from build123d import *

# Parameters (mm, degrees)
F1_DEPTH = 3.24


with BuildPart() as f1:
    # F0 (on Top) → F1 (new body)
    with BuildSketch(Plane.XY):
        Polygon((32.101754, 47.657341), (8.328551, 29.566584), (8.328551, 13.494031), (8.328551, 9.566584), (8.328551, 5.849354), (8.328551, -10.433416), (32.101754, 7.657341), align=None)
        Polygon((8.328551, 9.566584), (8.328551, 13.494031), (1.83994, 13.494031), (1.83994, 5.849354), (8.328551, 5.849354), align=None)
    extrude(amount=F1_DEPTH)


solid = f1.part
Part model, mm, in its own coordinate system. A direction names the side the tool comes from. Coordinates: 2 decimals unless noted, no trailing zeros. Write each loop counter-clockwise with the first axis right and the second up, starting at its lowest first coordinate (ties: lowest second). Pieces come first, ordered by that corner, then holes. Notation, with made-up numbers: M -1,-25.5 L 55,-25.5 A12 ccw 55,-10.5 Z; hole C -17.5,79.5 d5. An arc over 180 degrees is marked long. Return JSON: item names as keys, results as strings.
1. Saw through at B-B, the plane x = 4. Write the cut outline in (y, z).
Determined:
{"outline": "M 5.85,0 L 13.49,0 L 13.49,3.24 L 5.85,3.24 Z"}
2. Saw through at C-C, the plane y = 25. Write the cut outline in (x, z), then the cut area to 3 significant figures.
Determined:
{"outline": "M 8.33,0 L 32.1,0 L 32.1,3.24 L 8.33,3.24 Z", "area": "77.0 mm²"}
3. Saw through at A-A, the plane z = 1.8. Write the cut outline in (x, y), then the cut area to 3 significant figures.
Determined:
{"outline": "M 1.84,5.85 L 8.33,5.85 L 8.33,-10.43 L 32.1,7.66 L 32.1,47.66 L 8.33,29.57 L 8.33,13.49 L 1.84,13.49 Z", "area": "1,000 mm²"}
4. Probe L1, parallel to X at y = 22, z = 2.65; L2, parallel to Y at x = 7, z = 2; L3, parallel to Y at x = 19, z = 3.15. List the from-to ranges inside material, lowest first.
Determined:
{"L1": "8.33 to 32.1", "L2": "5.85 to 13.49", "L3": "-2.31 to 37.69"}
5. Flat gauge pins, fed straight in: pin 1 Ø1 at (x, z) = (20.5, 1) entering from +Y; pin 2 Ø1.6 at (y, z) = (24, 2) entering from -X; pin 3 Ø1 at (x, z) = (5.5, 1.5) entering from -Y. Where does each tip first touch, or does it go through?
Determined:
{"pin 1": "y = 39.21", "pin 2": "x = 8.33", "pin 3": "y = 5.85"}
6. 3-axis set-ups, long thin cutter, end or side, ignore diameter. For faces 1 (the face through (20.049, -1.515, 1.597)), 2 (the face through (5, 13.494, 2)), 3 (the face through (8.329, -2, 2)): which of +Z, -Z, +X, -X, +Y, -Y reach the whole face in a straight line?
Determined:
{"face 1": "+Z, -Z, +X, -Y", "face 2": "+Z, -Z, -X, +Y", "face 3": "+Z, -Z, -X, -Y"}
